The model under review builds one solid part; all positions refer to its coordinate system, in mm. Give positions to 0.01 mm unless a question says otherwise; leave off trailing zeros. Write each loop counter-clockwise with the first axis right and the second up, starting at its lowest first coordinate (ties: lowest second). Pieces come first, ordered by that corner, then holes. Notation, with made-up numbers: (-13.75, 46) - (-7.75, 46) arc R26 ccw to (-7.75, 83) - close; hole circle Ø4 at (74.25, 59). An arc over 180 degrees is marked (long way). One line per question, with ' | ' between items. Start each with the question number.
```python
from build123d import *

# Parameters (mm, degrees)
SKIZZE1_W                       = 120
SKIZZE1_H                       = 60
AUFSATZ_LINEAR_AUSTRAGEN1_DEPTH = 10
M6_GEWINDEBOHRUNG1_D            = 5
M5_GEWINDEBOHRUNG1_D            = 4.2
M4_GEWINDEBOHRUNG1_D            = 3.3


with BuildPart() as part:
    # Skizze1 → Aufsatz-Linear austragen1 (new body)
    with BuildSketch(Plane.XY):
        Rectangle(SKIZZE1_W, SKIZZE1_H)
    extrude(amount=AUFSATZ_LINEAR_AUSTRAGEN1_DEPTH)

    # M6 Gewindebohrung1 (through all)
    with Locations(Plane.XY.offset(10)):
        with Locations((-55, -25), (-55, 25), (55, 25), (55, -25)):
            Hole(M6_GEWINDEBOHRUNG1_D / 2)

    # M5 Gewindebohrung1 (through all)
    with Locations(Plane.XY.offset(10)):
        with Locations((-42, 0), (42, 0)):
            Hole(M5_GEWINDEBOHRUNG1_D / 2)

    # M4 Gewindebohrung1 (through all)
    with Locations(Plane.XY.offset(10)):
        with Locations((0, 3), (-15, -22), (15, -22)):
            Hole(M4_GEWINDEBOHRUNG1_D / 2)


solid = part.part
```
Item 1: Take a section at A-A (x = -15). Give the boundary of the cut face in (y, z), plus the area to 3 significant figures.
Item 2: Take a section at B-B (y = -25). Give the boundary of the cut face in (x, z), plus the area to 3 significant figures.
Item 3: For probe 1 along Y at (x, z) = (-55, 4.25); probe 2 along Y at (x, z) = (15, 4.25); probe 3 along X at (y, z) = (23.5, 9), list the stretches that pass through material, from the lowest coordinate up.
Item 4: Take a section at C-C (z = 8.25). State how many separate pieces and enclosed holes the cut face has, plus the area to 3 significant figures.
Item 5: Clearance check with a flat-ended pin moving along its axis: P1, Ø2, axis at x = 15, y = -22, coming from the -Z side. State where the tip first meets the part, or that it passes through.
Item 6: The part is to be moulded in two halves that separate along X. For faces 1 (the cylindrical face through (-56.34, 27.11, 4.93)), 2 (the flat face through (-1, 0, 10)), 3 (the flat face through (-60, 0, 5)), 4 (the cylindrical face through (-15.89, -20.61, 4.93)), say which applies: +X half, -X half, draft (parallel to the pull), parting line (faces both ways), or undercut.
Item 7: Take a section at D-D (x = 55). Give the boundary of the cut face in (y, z).
Check sheet entries:
1) outline: (-30, 0) - (-23.65, 0) - (-23.65, 10) - (-30, 10) - close; (-20.35, 0) - (30, 0) - (30, 10) - (-20.35, 10) - close | area: 567 mm^2
2) outline: (-60, 0) - (-57.5, 0) - (-57.5, 10) - (-60, 10) - close; (-52.5, 0) - (52.5, 0) - (52.5, 10) - (-52.5, 10) - close; (57.5, 0) - (60, 0) - (60, 10) - (57.5, 10) - close | area: 1,100 mm^2
3) probe 1: y = -30 to -27.5, -22.5 to 22.5, 27.5 to 30 | probe 2: y = -30 to -23.65, -20.35 to 30 | probe 3: x = -60 to -57, -53 to 53, 57 to 60
4) separate pieces: 1 | enclosed holes: 9 | area: 7,070 mm^2
5) P1: passes through
6) face 1: undercut | face 2: draft | face 3: -X half | face 4: undercut
7) outline: (-30, 0) - (-27.5, 0) - (-27.5, 10) - (-30, 10) - close; (-22.5, 0) - (22.5, 0) - (22.5, 10) - (-22.5, 10) - close; (27.5, 0) - (30, 0) - (30, 10) - (27.5, 10) - close
